Read the model definition and answer for the solid it produces. Units are mm, in the model's axes. A direction names the side the tool comes from. Give positions to 0.01 mm unless a question says otherwise; leave off trailing zeros. Write each loop counter-clockwise with the first axis right and the second up, starting at its lowest first coordinate (ties: lowest second). Pieces come first, ordered by that corner, then holes. Notation, with made-up numbers: (11, 73.5) -> (54, 73.5) arc R5 cw to (54, 78.5) -> close; hole circle Ø11 at (-32, 41). An arc over 180 degrees is marked (long way). Use a Markdown table: item, result.
Autodesk Inventor part; units mm, degrees
ref_plane "YZ Plane" through (0, 0, 0) normal (1, 0, 0) x (0, 1, 0)
ref_plane "XZ Plane" through (0, 0, 0) normal (0, 1, 0) x (-1, 0, 0)
ref_plane "XY Plane" through (0, 0, 0) normal (0, 0, 1) x (1, 0, 0)
sketch "Motor_Lego_Axle_Connector" plane through (0, 0, 0) normal (0, 0, 1) x (1, 0, 0)
  circle A0 centre (0, 0) radius 3.5
  circle A1 centre (0, 0) radius 2.7
  line L0 (-1.8, 2.0125) -> (-1.8, -2.0125)
  line L1 (0, 3.5) -> (0, -3.5) construction
  line L2 (1.8, 2.0125) -> (1.8, -2.0125)
  line L3 (0.9, 2.4) -> (-0.9, 2.4)
  line L4 (0.9, 2.4) -> (0.9, 1.4)
  line L5 (1.4, 1.4) -> (0.9, 1.4) construction
  line L6 (1.4, 1.4) -> (1.4, 0.9) construction
  arc A2 (0.9, 1.4) -> (1.4, 0.9) centre (1.4, 1.4) ccw
  line L7 (1.4, 0.9) -> (2.4, 0.9)
  line L8 (-0.9, 1.4) -> (-0.9, 2.4)
  arc A3 (-1.4, 0.9) -> (-0.9, 1.4) centre (-1.4, 1.4) ccw
  line L9 (-2.4, 0.9) -> (-1.4, 0.9)
  line L10 (-2.4, 0.9) -> (-2.4, -0.9)
  line L11 (-1.4, -0.9) -> (-2.4, -0.9)
  arc A4 (-0.9, -1.4) -> (-1.4, -0.9) centre (-1.4, -1.4) ccw
  line L12 (-0.9, -2.4) -> (-0.9, -1.4)
  line L13 (-0.9, -2.4) -> (0.9, -2.4)
  line L14 (0.9, -1.4) -> (0.9, -2.4)
  arc A5 (1.4, -0.9) -> (0.9, -1.4) centre (1.4, -1.4) ccw
  line L15 (2.4, -0.9) -> (1.4, -0.9)
  line L16 (2.4, -0.9) -> (2.4, 0.9)
  point P0 (1.8, -2.0125)
  point P1 (0, 2.4)
  point P2 (-2.4, 0)
  point P3 (0, -2.4)
  point P4 (2.4, 0)
  dimension "d0" = 7
  dimension "d1" = 5.4
  dimension "d2" = 7
  dimension "d3" = 1.8
  dimension "d12" = 1.8
  dimension "d13" = 2.4
  dimension "d14" = 1
  dimension "d16" = 0.5
  dimension "d17" = 1
  dimension "d20" = 360
extrude "Motor_Side_Outer_Ring_Extrusion" add sketch "Motor_Lego_Axle_Connector" along normal blind 9
extrude "Motor_Connector_Extrusion" add sketch "Motor_Lego_Axle_Connector" along normal blind 7.9 separate body contours A1 L2 L15 L16 L7 | L0 L9 L10 L11 A1 | L7 L16 L15 L2 | L0 L11 L10 L9
extrude "Seperation_Extrusion" add sketch "Motor_Lego_Axle_Connector" against normal blind 3 contours A1 L2 L15 L16 L7 | L2 L7 A2 L4 L3 L8 A3 L9 L0 A1 | A1 L0 L11 A4 L12 L13 L14 A5 L15 L2 | L0 L9 L10 L11 A1 | L7 L16 L15 L2 | L2 L15 A5 L14 L13 L12 A4 L11 L0 L9 A3 L8 L3 L4 A2 L7 | L0 L11 L10 L9
extrude "Lego_Axle_Side_Outer_Ring_Extrusion" add sketch "Motor_Lego_Axle_Connector" against normal blind 11
extrude "Lego_Axle_Connector_Extrusion" add sketch "Motor_Lego_Axle_Connector" against normal blind 11 contours A1 L2 L15 L16 L7 | L2 L7 A2 L4 L3 L8 A3 L9 L0 A1 | A1 L0 L11 A4 L12 L13 L14 A5 L15 L2 | L0 L9 L10 L11 A1
equation "\"d2\" = d0"
properties part number "Motor_Lego_Axle_Connector"
Item 1: A tool of negligible diameter and unlimited length cuts with its end or side. For faces 4 (the face through (2, 0, 7.9)), 5 (the face through (2, -2, -11)), 6 (the face through (0, 0, -3)), from which of +Z, -Z, +X, -X, +Y, -Y can it reach the whole face along a straight path? Write none if from no direction.
Return value:
| item | result |
|---|---|
| face 4 | +Z |
| face 5 | -Z, +X, -X, +Y, -Y |
| face 6 | -Z |
Item 2: A cutting plane is placed at A-A (z = -9.5). Give the vertices of the cut face in (x, y), then the cut area to 3 significant figures.
Return value:
| item | result |
|---|---|
| outline | circle Ø7 at (0, 0); hole (-2.4, -0.9) -> (-1.4, -0.9) arc R0.5 cw to (-0.9, -1.4) -> (-0.9, -2.4) -> (0.9, -2.4) -> (0.9, -1.4) arc R0.5 cw to (1.4, -0.9) -> (2.4, -0.9) -> (2.4, 0.9) -> (1.4, 0.9) arc R0.5 cw to (0.9, 1.4) -> (0.9, 2.4) -> (-0.9, 2.4) -> (-0.9, 1.4) arc R0.5 cw to (-1.4, 0.9) -> (-2.4, 0.9) -> close |
| area | 24.2 mm^2 |
Item 3: A cutting plane is placed at D-D (z = 2). Give the vertices of the cut face in (x, y).
Return value:
| item | result |
|---|---|
| outline | circle Ø7 at (0, 0); hole (-1.8, -2.01) arc R2.7 ccw to (1.8, -2.01) -> (1.8, 2.01) arc R2.7 ccw to (-1.8, 2.01) -> close |
Item 4: For a pull along X with two mould halves and no side action, classify faces 1 (the face through (1, -3, 9)), 2 (the face through (-2.4, 0, -7)), 3 (the face through (3.233, -1.341, -0.86)) as +X half, -X half, draft (parallel to the pull), parting line (faces both ways), or undercut.
Return value:
| item | result |
|---|---|
| face 1 | draft |
| face 2 | undercut |
| face 3 | parting line |
Item 5: Straight lines are drawn through the part: line 1 along Y through (x, z) = (0, -5.25); line 2 along Z through (x, y) = (0.5, -2.5); line 3 along Y through (x, z) = (0, 2.5). For each, find the intervals that lie inside material, in ascending order. Write a range as [from, to].
Return value:
| item | result |
|---|---|
| line 1 | [-3.5, -2.4], [2.4, 3.5] |
| line 2 | [-11, 0] |
| line 3 | [-3.5, -2.7], [2.7, 3.5] |
Item 6: Each of these flat-tipped pins is pushed along its axis until it touches: P1, Ø0.5, axis at x = -0.5, z = -7, coming from the -Y side; P2, Ø4, axis at x = 2, y = -1, coming from the +Z side; P3, Ø0.8, axis at y = 2, z = -9, coming from the +X side; P4, Ø0.5, axis at x = -2, z = -7.5, coming from the +Y side. Where does it stop, or does it pass through?
Return value:
| item | result |
|---|---|
| P1 | y = -3.49 |
| P2 | z = 9 |
| P3 | x = 3.11 |
| P4 | y = 3.03 |
Item 7: A cutting plane is placed at C-C (x = 0). Give the vertices of the cut face in (y, z), then the cut area to 3 significant figures.
Return value:
| item | result |
|---|---|
| outline | (-3.5, -11) -> (-2.4, -11) -> (-2.4, -3) -> (2.4, -3) -> (2.4, -11) -> (3.5, -11) -> (3.5, 9) -> (2.7, 9) -> (2.7, 0) -> (-2.7, 0) -> (-2.7, 9) -> (-3.5, 9) -> close |
| area | 53.0 mm^2 |
Item 8: A cutting plane is placed at B-B (y = 0). Give the vertices of the cut face in (x, z).
Return value:
| item | result |
|---|---|
| outline | (-3.5, -11) -> (-2.4, -11) -> (-2.4, -3) -> (2.4, -3) -> (2.4, -11) -> (3.5, -11) -> (3.5, 9) -> (2.7, 9) -> (2.7, 7.9) -> (1.8, 7.9) -> (1.8, 0) -> (-1.8, 0) -> (-1.8, 7.9) -> (-2.7, 7.9) -> (-2.7, 9) -> (-3.5, 9) -> close |
